Can you work these out from the model? Positions are in its coordinate system, mm. Coordinates: 2 decimals unless noted, no trailing zeros.
```python
from build123d import *

# Parameters (mm, degrees)
BOSS_EXTRUDE1_DEPTH = 914.4
CUT_EXTRUDE1_DEPTH  = 1.778
LPATTERN1_COUNT     = 18
LPATTERN1_PITCH     = 50.8


with BuildPart() as part:
    # Sketch1 → Boss-Extrude1 (new body)
    with BuildSketch(Plane.XY):
        with BuildLine():
            Line((-15.58925, 20.6375), (-3.46075, 20.6375))
            ThreePointArc((-3.46075, 20.6375), (-1.013630207, 19.623869793), (0, 17.17675))
            Line((0, 17.17675), (0, -17.17675))
            ThreePointArc((0, -17.17675), (-1.013630207, -19.623869793), (-3.46075, -20.6375))
            Line((-3.46075, -20.6375), (-15.58925, -20.6375))
            ThreePointArc((-15.58925, -20.6375), (-19.158901808, -19.158901808), (-20.6375, -15.58925))
            Line((-20.6375, -15.58925), (-20.6375, -14.57325))
            ThreePointArc((-20.6375, -14.57325), (-19.623869793, -12.126130207), (-17.17675, -11.1125))
            Line((-17.17675, -11.1125), (-14.3891, -11.1125))
            ThreePointArc((-14.3891, -11.1125), (-13.5001, -12.0015), (-14.3891, -12.8905))
            Line((-14.3891, -12.8905), (-17.17675, -12.8905))
            ThreePointArc((-17.17675, -12.8905), (-18.366633936, -13.383366064), (-18.8595, -14.57325))
            Line((-18.8595, -14.57325), (-18.8595, -15.58925))
            ThreePointArc((-18.8595, -15.58925), (-17.901665951, -17.901665951), (-15.58925, -18.8595))
            Line((-15.58925, -18.8595), (-3.46075, -18.8595))
            ThreePointArc((-3.46075, -18.8595), (-2.270866064, -18.366633936), (-1.778, -17.17675))
            Line((-1.778, -17.17675), (-1.778, 17.17675))
            ThreePointArc((-1.778, 17.17675), (-2.270866064, 18.366633936), (-3.46075, 18.8595))
            Line((-3.46075, 18.8595), (-15.58925, 18.8595))
            ThreePointArc((-15.58925, 18.8595), (-17.901665951, 17.901665951), (-18.8595, 15.58925))
            Line((-18.8595, 15.58925), (-18.8595, 14.57325))
            ThreePointArc((-18.8595, 14.57325), (-18.366633936, 13.383366064), (-17.17675, 12.8905))
            Line((-17.17675, 12.8905), (-14.3891, 12.8905))
            ThreePointArc((-14.3891, 12.8905), (-13.5001, 12.0015), (-14.3891, 11.1125))
            Line((-14.3891, 11.1125), (-17.17675, 11.1125))
            ThreePointArc((-17.17675, 11.1125), (-19.623869793, 12.126130207), (-20.6375, 14.57325))
            Line((-20.6375, 14.57325), (-20.6375, 15.58925))
            ThreePointArc((-20.6375, 15.58925), (-19.158901808, 19.158901808), (-15.58925, 20.6375))
        make_face()
    extrude(amount=-BOSS_EXTRUDE1_DEPTH)

    # Sketch2 → Cut-Extrude1 (cut)
    with BuildSketch(Plane(origin=(0, 0, 0), x_dir=(0, 0, -1), z_dir=(1, 0, 0))):
        with BuildLine():
            Line((18.25625, 7.14375), (32.54375, 7.14375))
            ThreePointArc((32.54375, 7.14375), (39.6875, 0), (32.54375, -7.14375))
            Line((32.54375, -7.14375), (18.25625, -7.14375))
            ThreePointArc((18.25625, -7.14375), (11.1125, 0), (18.25625, 7.14375))
        make_face()
    cut_extrude1 = extrude(amount=-CUT_EXTRUDE1_DEPTH, mode=Mode.SUBTRACT)

    # LPattern1: Cut-Extrude1 ×18
    with Locations(*[(0, 0, -i * LPATTERN1_PITCH) for i in range(1, LPATTERN1_COUNT)]):
        add(cut_extrude1, mode=Mode.SUBTRACT)


solid = part.part
```
1. I'm going to push flat-ended pins straight in: pin 1 (1.4 mm diameter, centred on x = -1, z = -535, fed in from +Y); pin 2 (1.4 mm diameter, centred on x = -1, z = -483, fed in from -Y); pin 3 (2 mm diameter, centred on x = -1, z = -231.5, fed in from +Y). Where does each tip first touch, or does it pass through?
Completed:
pin 1: stops at y = 20.16
pin 2: stops at y = -20.16
pin 3: stops at y = 20.31
2. Thinking about a two-plate mould opening in X: for faces 1 (the flat face through (0, 0, -451)), 2 (the flat face through (-1.778, 0, -451)), 3 (the flat face through (-1, 0, 0)), which applies, pulls with the +X half, pulls with the -X half, needs draft (parallel to the pull), parting line crosses it, or undercut?
Completed:
face 1: pulls with the +X half
face 2: undercut
face 3: needs draft
3. Imagine slicing it at A-A on y = 0. Give the number of separate pieces and of enclosed holes in the cut face, then the cut area to 3 significant figures.
Completed:
separate pieces: 19
enclosed holes: 0
area: 711 mm2
4. Please list where these lines run through material, in increasing order: probe 1 along X at (y, z) = (11.5, -145); probe 2 along Y at (x, z) = (-18.5, -373); probe 3 along Y at (x, z) = (-7.5, -102).
Completed:
probe 1: x = -18.77 to -13.66, -1.78 to 0
probe 2: y = -19.71 to -17.08, -13.53 to -11.38, 11.38 to 13.53, 17.08 to 19.71
probe 3: y = -20.64 to -18.86, 18.86 to 20.64
